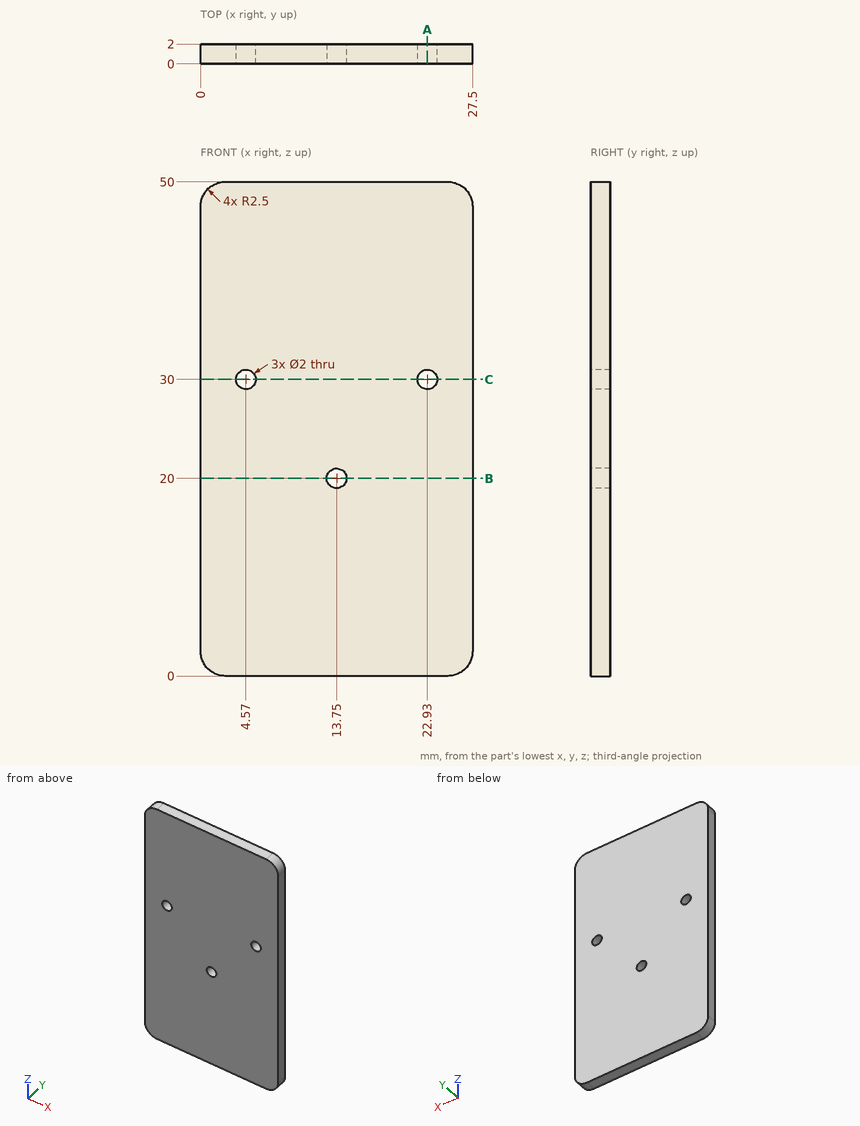
Verification items for this drawing (mm, ordinates from the low corner). Round coordinates to 2 decimals unless told otherwise and drop trailing zeros. Write each loop counter-clockwise with the first axis right and the second up, starting at its lowest first coordinate (ties: lowest second). Pieces come first, ordered by that corner, then holes. Notation, with made-up numbers: (23.5, -15.75) - (76.5, -15.75) arc R9 cw to (76.5, -4.75) - close; hole circle Ø3 at (64.25, 4). An arc over 180 degrees is marked (long way). Answer as a JSON object with one key per item and string values. Group by question number.
Q1. Section check B-B, the plane z = 20. Enter the section's corners in (x, y), plus the area to 3 significant figures.
Q2. Section check A-A, the plane x = 22.93. Enter the section's corners in (y, z).
Q3. Thickness scan on line 1 (X direction, y = 0.7, z = 30); line 2 (Z direction, x = 4.57, y = 0.85); line 3 (Z direction, x = 23.25, y = 0.75). Record the ranges inside material, lowest first.
Q4. Section check C-C, the plane z = 30. Enter the section's corners in (x, y), plus the area to 3 significant figures.
Found:
{
 "1": {"outline": "(0, 0) - (12.75, 0) - (12.75, 2) - (0, 2) - close; (14.75, 0) - (27.5, 0) - (27.5, 2) - (14.75, 2) - close", "area": "51.0 mm^2"},
 "2": {"outline": "(0, 0) - (2, 0) - (2, 29) - (0, 29) - close; (0, 31) - (2, 31) - (2, 50) - (0, 50) - close"},
 "3": {"line 1": "x = 0 to 3.57, 5.57 to 21.93, 23.93 to 27.5", "line 2": "z = 0 to 29, 31 to 50", "line 3": "z = 0 to 29.05, 30.95 to 50"},
 "4": {"outline": "(0, 0) - (3.57, 0) - (3.57, 2) - (0, 2) - close; (5.57, 0) - (21.93, 0) - (21.93, 2) - (5.57, 2) - close; (23.93, 0) - (27.5, 0) - (27.5, 2) - (23.93, 2) - close", "area": "47.0 mm^2"}
}
